For this review, take the finished solid that the model builds, in its own axes (mm). A direction names the side the tool comes from. Coordinates: 2 decimals unless noted, no trailing zeros. Loops run counter-clockwise (first coordinate to the right, second up) from the corner with the lowest first, then second, coordinate; pieces in that order, holes last. Notation, with made-up numbers: (78, 1) -> (82, 1) arc R37 ccw to (82, 39) -> close; hole circle Ø8 at (-22, 49.25). An arc over 180 degrees is marked (long way). Use a Markdown table: item, result.
from build123d import *

# Parameters (mm, degrees)
SKETCH_2_R          = 1.5
CUT_EXTRUDE_1_DEPTH = 16
SKETCH_4_OUTSIDE_W  = 74.818
SKETCH_4_OUTSIDE_H  = 74.818
CUT_EXTRUDE_3_DEPTH = 16


with BuildPart() as part:
    # 草图1 → 旋转1 (revolve)
    with BuildSketch(Plane.XY):
        Polygon((22, 1.5), (22, -15), (23, -15), (23, -2), (28.25, -2), (28.25, 0), (23, 0), (23, 1.5), align=None)
    revolve(axis=Axis((0, 0, 0), (0, 1, 0)))

    # 草图2 → 切除-拉伸1 (cut, through all)
    with BuildSketch(Plane(origin=(0, 0, 0), x_dir=(1, 0, 0), z_dir=(0, 1, 0))):
        with Locations((-18.207999616, 18.207999616)):
            Circle(SKETCH_2_R)
        with Locations((18.207999616, 18.207999616)):
            Circle(SKETCH_2_R)
        with Locations((18.207999616, -18.207999616)):
            Circle(SKETCH_2_R)
        with Locations((-18.207999616, -18.207999616)):
            Circle(SKETCH_2_R)
    extrude(amount=-CUT_EXTRUDE_1_DEPTH, mode=Mode.SUBTRACT)

    # 草图4 outside → 切除-拉伸3 (cut, through all)
    with BuildSketch(Plane(origin=(0, 0, 0), x_dir=(1, 0, 0), z_dir=(0, 1, 0))):
        Rectangle(SKETCH_4_OUTSIDE_W, SKETCH_4_OUTSIDE_H)
        with BuildLine():
            ThreePointArc((-16.199808887, 19.697016069), (-19.975766569, 19.975766569), (-19.697016069, 16.199808887))
            ThreePointArc((-19.697016069, 16.199808887), (-18.722615608, 14.617736813), (-19.10897051, 12.800283045))
            ThreePointArc((-19.10897051, 12.800283045), (-23, 0), (-19.10897051, -12.800283045))
            ThreePointArc((-19.10897051, -12.800283045), (-18.722615608, -14.617736813), (-19.697016069, -16.199808887))
            ThreePointArc((-19.697016069, -16.199808887), (-19.975766569, -19.975766569), (-16.199808887, -19.697016069))
            ThreePointArc((-16.199808887, -19.697016069), (-14.617736813, -18.722615608), (-12.800283045, -19.10897051))
            ThreePointArc((-12.800283045, -19.10897051), (0, -23), (12.800283045, -19.10897051))
            ThreePointArc((12.800283045, -19.10897051), (14.617736813, -18.722615608), (16.199808887, -19.697016069))
            ThreePointArc((16.199808887, -19.697016069), (19.975766569, -19.975766569), (19.697016069, -16.199808887))
            ThreePointArc((19.697016069, -16.199808887), (18.722615608, -14.617736813), (19.10897051, -12.800283045))
            ThreePointArc((19.10897051, -12.800283045), (23, 0), (19.10897051, 12.800283045))
            ThreePointArc((19.10897051, 12.800283045), (18.722615608, 14.617736813), (19.697016069, 16.199808887))
            ThreePointArc((19.697016069, 16.199808887), (19.975766569, 19.975766569), (16.199808887, 19.697016069))
            ThreePointArc((16.199808887, 19.697016069), (14.617736813, 18.722615608), (12.800283045, 19.10897051))
            ThreePointArc((12.800283045, 19.10897051), (0, 23), (-12.800283045, 19.10897051))
            ThreePointArc((-12.800283045, 19.10897051), (-14.617736813, 18.722615608), (-16.199808887, 19.697016069))
        make_face(mode=Mode.SUBTRACT)
    extrude(amount=-CUT_EXTRUDE_3_DEPTH, mode=Mode.SUBTRACT)


solid = part.part
(1) For line 1 along X through (y, z) = (-4.75, 0.5); line 2 along Z through (x, y) = (-2, -6.5), list the stretches that pass through material, from the lowest coordinate up.
Found:
| item | result |
|---|---|
| line 1 | x = -22.99 to -21.99, 21.99 to 22.99 |
| line 2 | z = -22.91 to -21.91, 21.91 to 22.91 |
(2) Take a section at C-C on y = -9.25. Write out the cut boundary in (x, z).
Found:
| item | result |
|---|---|
| outline | circle Ø46 at (0, 0); hole circle Ø44 at (0, 0) |
(3) Take a section at D-D on z = 13.5. Write out the cut boundary in (x, y).
Found:
| item | result |
|---|---|
| outline | (-18.78, -2) -> (-18.62, -2) -> (-18.62, -15) -> (-17.37, -15) -> (-17.37, 1.5) -> (-18.62, 1.5) -> (-18.62, 0) -> (-18.78, 0) -> close; (17.37, -15) -> (18.62, -15) -> (18.62, -2) -> (18.78, -2) -> (18.78, 0) -> (18.62, 0) -> (18.62, 1.5) -> (17.37, 1.5) -> close |
(4) Mouldability with a two-part tool opening along Z and no side actions: class faces 1 (the face through (17, 0, -17)), 2 (the face through (-4.769, -6.866, 21.477)) as pulls with the +Z half, pulls with the -Z half, needs draft (parallel to the pull), parting line crosses it, or undercut.
Found:
| item | result |
|---|---|
| face 1 | needs draft |
| face 2 | undercut |
(5) Take a section at A-A on z = -2.5. Write out the cut boundary in (x, y).
Found:
| item | result |
|---|---|
| outline | (-22.86, -15) -> (-21.86, -15) -> (-21.86, 1.5) -> (-22.86, 1.5) -> close; (21.86, -15) -> (22.86, -15) -> (22.86, 1.5) -> (21.86, 1.5) -> close |
(6) For pin 1 Ø6.5 at (x, z) = (18.5, -18.5) entering from -Y; pin 2 Ø8 at (y, z) = (-9.5, 11.5) entering from -X; pin 3 Ø4 at (x, z) = (18.208, 18.208) entering from -Y; pin 4 Ø2 at (y, z) = (-0.5, 6) entering from +X, all flat-tipped, find the tip position at first contact; note any pin that passes through.
Found:
| item | result |
|---|---|
| pin 1 | stops at y = -15 |
| pin 2 | stops at x = -21.74 |
| pin 3 | stops at y = -2 |
| pin 4 | stops at x = 22.45 |
(7) For faces 3 (the face through (-17, -2, 17)), 4 (the face through (-18.533, -0.986, 19.672)), 5 (the face through (17, -2, 17)), 6 (the face through (17, 0, 17)), 7 (the face through (-17, -2, -17)), list the 3-axis set-ups (+Z, -Z, +X, -X, +Y, -Y) from which the entire face can be reached by the end or side of a thin tool; tool diameter is ignored.
Found:
| item | result |
|---|---|
| face 3 | +Z, -X, -Y |
| face 4 | +Y, -Y |
| face 5 | +Z, +X, -Y |
| face 6 | +Z, +X, +Y |
| face 7 | -Z, -X, -Y |
(8) Take a section at B-B on x = 4. Write out the cut boundary in (y, z).
Found:
| item | result |
|---|---|
| outline | (-15, -22.65) -> (1.5, -22.65) -> (1.5, -21.63) -> (-15, -21.63) -> close; (-15, 21.63) -> (1.5, 21.63) -> (1.5, 22.65) -> (-15, 22.65) -> close |
